```python
from build123d import *

# Parameters (mm, degrees)
BOSS_EXTRUDE1_DEPTH   = 20
CUT_EXTRUDE1_DEPTH    = 10
SKETCH3_R             = 10
CUT_EXTRUDE2_DEPTH    = 210.276793028
SKETCH4_R             = 5
CUT_EXTRUDE3_DEPTH    = 210.992323907
CRVPATTERN1_START     = -20
CRVPATTERN1_OUTLINE_R = 5
CRVPATTERN1_DEPTH     = 20


# Read off the part's stored shape, not the designer's step: CrvPattern1
with BuildPart() as part:
    # Sketch1 → Boss-Extrude1 (new body)
    with BuildSketch(Plane.XY):
        with BuildLine():
            Line((0, 96), (89.69, 96))
            ThreePointArc((89.69, 96), (185.69, 0), (89.69, -96))
            Line((89.69, -96), (0, -96))
            ThreePointArc((0, -96), (-96, 0), (0, 96))
        make_face()
    extrude(amount=-BOSS_EXTRUDE1_DEPTH)

    # Sketch2 → Cut-Extrude1 (cut)
    with BuildSketch(Plane.XY):
        with BuildLine():
            ThreePointArc((44.845, 53.422733691), (-69.75, 0), (44.845, -53.422733691))
            ThreePointArc((44.845, -53.422733691), (159.44, 0), (44.845, 53.422733691))
        make_face()
    extrude(amount=-CUT_EXTRUDE1_DEPTH, mode=Mode.SUBTRACT)

    # Sketch3 → Cut-Extrude2 (cut, through all)
    with BuildSketch(Plane.XY.offset(-10)):
        Circle(SKETCH3_R)
        with Locations((89.69, 0)):
            Circle(SKETCH3_R)
    extrude(amount=-CUT_EXTRUDE2_DEPTH, mode=Mode.SUBTRACT)

    # Sketch4 → Cut-Extrude3 (cut, through all)
    with BuildSketch(Plane.XY):
        with Locations((172.565, 0)):
            Circle(SKETCH4_R)
    extrude(amount=-CUT_EXTRUDE3_DEPTH, mode=Mode.SUBTRACT)

    # CrvPattern1 outline → CrvPattern1 (cut)
    with BuildSketch(Plane.XY.offset(CRVPATTERN1_START)):
        with Locations((160.625248894, 42.853892348)):
            Circle(CRVPATTERN1_OUTLINE_R)
        with Locations((160.625248894, -42.853892348)):
            Circle(CRVPATTERN1_OUTLINE_R)
        with Locations((128.24630101, -73.359916013)):
            Circle(CRVPATTERN1_OUTLINE_R)
        with Locations((83.973289474, -82.875)):
            Circle(CRVPATTERN1_OUTLINE_R)
        with Locations((31.802236842, -82.875)):
            Circle(CRVPATTERN1_OUTLINE_R)
        with Locations((-17.452379652, -81.01654195)):
            Circle(CRVPATTERN1_OUTLINE_R)
        with Locations((-56.830926836, -60.320074436)):
            Circle(CRVPATTERN1_OUTLINE_R)
        with Locations((-79.834279533, -22.243053668)):
            Circle(CRVPATTERN1_OUTLINE_R)
        with Locations((-79.834279533, 22.243053668)):
            Circle(CRVPATTERN1_OUTLINE_R)
        with Locations((-56.830926836, 60.320074436)):
            Circle(CRVPATTERN1_OUTLINE_R)
        with Locations((-17.452379652, 81.01654195)):
            Circle(CRVPATTERN1_OUTLINE_R)
        with Locations((31.802236842, 82.875)):
            Circle(CRVPATTERN1_OUTLINE_R)
        with Locations((83.973289474, 82.875)):
            Circle(CRVPATTERN1_OUTLINE_R)
        with Locations((128.24630101, 73.359916013)):
            Circle(CRVPATTERN1_OUTLINE_R)
    extrude(amount=CRVPATTERN1_DEPTH, mode=Mode.SUBTRACT)


solid = part.part
```
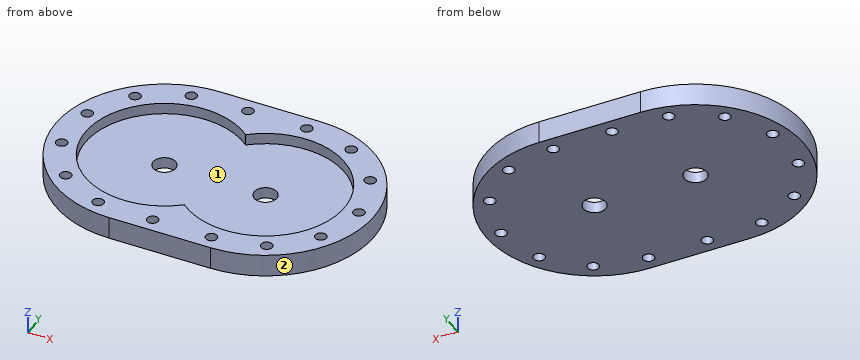
Source: CAD feature listing. Evaluate the final solid. Frame: model axes, mm. Face numbers are marked on the shaded views. A direction names the side the tool comes from. Round coordinates to 2 decimals unless told otherwise and drop trailing zeros. Write each loop counter-clockwise with the first axis right and the second up, starting at its lowest first coordinate (ties: lowest second). Pieces come first, ordered by that corner, then holes. Notation, with made-up numbers: M 6,26 L 63,26 A12 cw 63,48 Z; hole C 44,9 d10. An arc over 180 degrees is marked long. Answer as a JSON object with one key per item and string values. Group by question number.
(1) Ray query, line 1 (Y direction, x = 89.69, z = -5); line 2 (X direction, y = -64, z = -5); line 3 (Y direction, x = 84, z = -4). Return the intervals inside material, ascending. Write a range as [from, to].
(2) Section query A-A on y = 0. Output: boundary loops of the cut face in (x, z) (3 decimals), then the cut area to 3 significant figures.
(3) Section query D-D on y = 34. Output: boundary loops of the cut face in (x, z).
(4) First-contact query: pin 1 (16 mm diameter, centred on x = 31.8, y = 82.88, fed in from +Z); pin 2 (4 mm diameter, centred on y = 32.5, z = -18, fed in from -X); pin 3 (4 mm diameter, centred on x = 139.5, z = -7, fed in from +Y); pin 4 (5 mm diameter, centred on x = -9.5, z = -3.5, fed in from -Y). Flat tips, straight axial feed; report the tip coordinate or a pass-through.
(5) Section query B-B on x = 106. Output: boundary loops of the cut face in (y, z), then the cut area to 3 significant figures.
(6) Reachability of the marked faces 1 and 2 from +Z, -Z, +X, -X, +Y, -Y: full face, straight path, thin tool, end or side. Return the list, or none.
(7) Section query C-C on z = -6. State how many separate pieces and enclosed holes the cut face has, then the cut area to 3 significant figures.
Computed values:
{
 "1": {"line 1": "[-96, -69.75], [69.75, 96]", "line 2": "[-71.55, -60.22], [-53.45, -27.73], [27.73, 61.96], [117.42, 161.24]", "line 3": "[-96, -87.87], [-77.88, -69.52], [69.52, 77.88], [87.87, 96]"},
 "2": {"outline": "M -96,-20 L -10,-20 L -10,-10 L -69.75,-10 L -69.75,0 L -96,0 Z; M 10,-20 L 79.69,-20 L 79.69,-10 L 10,-10 Z; M 99.69,-20 L 167.565,-20 L 167.565,0 L 159.44,0 L 159.44,-10 L 99.69,-10 Z; M 177.565,-20 L 185.69,-20 L 185.69,0 L 177.565,0 Z", "area": "2,740 mm^2"},
 "3": {"outline": "M -89.78,-20 L 179.47,-20 L 179.47,0 L 150.59,0 L 150.59,-10 L -60.9,-10 L -60.9,0 L -89.78,0 Z"},
 "4": {"pin 1": "z = 0", "pin 2": "x = -91.03", "pin 3": "y = 83.25", "pin 4": "y = -95.74"},
 "5": {"outline": "M -94.6,-20 L 94.6,-20 L 94.6,0 L 67.82,0 L 67.82,-10 L -67.82,-10 L -67.82,0 L -94.6,0 Z", "area": "2,430 mm^2"},
 "6": {"face 1": "+Z", "face 2": "+Z, -Z, +X"},
 "7": {"separate pieces": "1", "enclosed holes": "16", "area": "18,100 mm^2"}
}
